Work out the finished part from the listing and answer in its coordinate system (mm). A direction names the side the tool comes from. Give positions to 0.01 mm unless a question says otherwise; leave off trailing zeros. Loops run counter-clockwise (first coordinate to the right, second up) from the corner with the lowest first, then second, coordinate; pieces in that order, holes last. Notation, with made-up numbers: M 68.5,73 L 85.5,73 A13 cw 85.5,77 Z; hole C 1.25,2.5 d4. An arc over 180 degrees is marked long. Answer as a JSON object with one key per item and string values. Group by question number.
Autodesk Inventor part; units mm, degrees
ref_plane "YZ Plane" through (0, 0, 0) normal (1, 0, 0) x (0, 1, 0)
ref_plane "XZ Plane" through (0, 0, 0) normal (0, 1, 0) x (-1, 0, 0)
ref_plane "XY Plane" through (0, 0, 0) normal (0, 0, 1) x (1, 0, 0)
sketch "Sketch1" plane through (0, 0, 0) normal (0, 0, 1) x (1, 0, 0)
  line L0 (0, 0) -> (0, 10)
  line L1 (0, 10) -> (60, 10)
  line L2 (60, 10) -> (60, 0)
  line L3 (0, 0) -> (7.5, 0)
  line L4 (7.5, 0) -> (7.5, -7.5)
  line L5 (7.5, -7.5) -> (-2.5, -7.5)
  line L6 (-2.5, -7.5) -> (-2.5, -17.5)
  line L7 (30, 10) -> (30, -7.5) construction
  line L8 (60, 0) -> (52.5, 0)
  line L9 (52.5, 0) -> (52.5, -7.5)
  line L10 (52.5, -7.5) -> (62.5, -7.5)
  line L11 (62.5, -7.5) -> (62.5, -17.5)
  line L12 (62.5, -17.5) -> (50.5, -17.5)
  line L13 (50.5, -17.5) -> (50.5, -37.5)
  line L14 (50.5, -37.5) -> (42.5, -37.5)
  line L15 (42.5, -37.5) -> (42.5, -17.5)
  line L16 (42.5, -17.5) -> (-2.5, -17.5)
  dimension "d0" = 10
  dimension "d2" = 60
  dimension "d3" = 7.5
  dimension "d4" = 7.5
  dimension "d5" = 10
  dimension "d6" = 10
  dimension "d21" = 12
  dimension "d22" = 20
  dimension "d23" = 8
extrude "Extrusion1" add sketch "Sketch1" along normal blind 12
sketch "Sketch2" plane through (50.5, -37.5, 0) normal (1, 0, 0) x (0, 0, -1)
  line L0 (0, 20) -> (0, 30)
  line L1 (0, 0) -> (0, 20)
  line L2 (-12, 0) -> (-12, 8)
  line L3 (0, 0) -> (-12, 0)
  line L4 (0, 0) -> (-6, 0)
  line L5 (-6, 0) -> (-6, 20)
  line L6 (-6, 20) -> (-6, 17)
  line L7 (-6, 17) -> (-6, 11)
  circle A0 centre (-6, 17) radius 1.5
  circle A1 centre (-6, 11) radius 1.5
  point P0 (0, 37.5)
  dimension "d24" = 6
  dimension "d27" = 3
  dimension "d28" = 6
  dimension "d29" = 3
  dimension "d30" = 3
extrude "Extrusion2" cut sketch "Sketch2" against normal through all
fillet "Fillet1" radius 2 1 edges at (-2.5, -17.5, 6)
properties part number "Basegripper" material "Copper, Wrought"
Item 1: A tool of negligible diameter and unlimited length cuts with its end or side. For faces 5 (the flat face through (60, 5, 6)), 6 (the flat face through (3, -7.5, 6)), 7 (the flat face through (42.5, -28, 5)), 8 (the flat face through (57, -7.5, 6)), 9 (the flat face through (57, -17.5, 6)), from which of +Z, -Z, +X, -X, +Y, -Y can it reach the whole face along a straight path? Write none if from no direction.
Item 2: Given pin 1 Ø3 at (x, y) = (12, -20) entering from +Z; pin 2 Ø6 at (y, z) = (-2, 4.5) entering from +X; pin 3 Ø6 at (x, z) = (54.5, 4.5) entering from -Y; pin 4 Ø5 at (y, z) = (-28.5, 5) entering from +X, each flat-ended and moving along its own axis, determine where each tip first touches the part or whether it passes through.
Item 3: A cutting plane is placed at D-D (x = 47). Determine the outline of the cut face in (y, z), and give its area (3 significant figures).
Item 4: A cutting plane is placed at A-A (z = 6). Determine the outline of the cut face in (x, y), and give its area (3 significant figures).
Item 5: Find the intervals of material crossed by probe 1 along Y at (x, z) = (45.5, 6); probe 2 along Y at (x, z) = (57, 6.25); probe 3 along Z at (x, y) = (47, -20.5), in increasing order. Write a range as [from, to].
Item 6: For a pull along Y with two mould halves and no side action, classify faces 1 (the flat face through (30, -3, 0)), 2 (the cylindrical face through (46.56, -19.49, 7.11)), 3 (the flat face through (21, -17.5, 6)), 4 (the flat face through (30, 10, 6)) as pulls with the +Y half, pulls with the -Y half, needs draft (parallel to the pull), parting line crosses it, or undercut.
Item 7: A cutting plane is placed at B-B (x = 53.5). Determine the outline of the cut face in (y, z).
Item 8: A cutting plane is placed at C-C (y = -26.5). Determine the outline of the cut face in (x, z), and give its area (3 significant figures).
The answers:
{
 "1": {"face 5": "+Z, -Z, +X, +Y", "face 6": "+Z, -Z, -X", "face 7": "+Z, -Z, -X, -Y", "face 8": "+Z, -Z, +X", "face 9": "+Z, -Z, +X, -Y"},
 "2": {"pin 1": "passes through", "pin 2": "stops at x = 60", "pin 3": "stops at y = -17.5", "pin 4": "stops at x = 50.5"},
 "3": {"outline": "M -37.5,0 L 10,0 L 10,12 L -37.5,12 Z; hole C -26.5,6 d3; hole C -20.5,6 d3", "area": "556 mm^2"},
 "4": {"outline": "M -2.5,-15.5 A2 ccw -0.5,-17.5 L 42.5,-17.5 L 42.5,-19 L 50.5,-19 L 50.5,-17.5 L 62.5,-17.5 L 62.5,-7.5 L 52.5,-7.5 L 52.5,0 L 60,0 L 60,10 L 0,10 L 0,0 L 7.5,0 L 7.5,-7.5 L -2.5,-7.5 Z; M 42.5,-37.5 L 50.5,-37.5 L 50.5,-28 L 42.5,-28 Z; M 42.5,-25 L 50.5,-25 L 50.5,-22 L 42.5,-22 Z", "area": "1,700 mm^2"},
 "5": {"probe 1": "y = [-37.5, -28], [-25, -22], [-19, 10]", "probe 2": "y = [-17.5, -7.5], [0, 10]", "probe 3": "z = [0, 4.5], [7.5, 12]"},
 "6": {"face 1": "needs draft", "face 2": "undercut", "face 3": "pulls with the -Y half", "face 4": "pulls with the +Y half"},
 "7": {"outline": "M -17.5,0 L -7.5,0 L -7.5,12 L -17.5,12 Z; M 0,0 L 10,0 L 10,12 L 0,12 Z"},
 "8": {"outline": "M 42.5,0 L 50.5,0 L 50.5,4.5 L 42.5,4.5 Z; M 42.5,7.5 L 50.5,7.5 L 50.5,12 L 42.5,12 Z", "area": "72.0 mm^2"}
}
